Part model, mm, in its own coordinate system. Face numbers are marked on the shaded views. A direction names the side the tool comes from. Round coordinates to 2 decimals unless told otherwise and drop trailing zeros. Write each loop counter-clockwise with the first axis right and the second up, starting at its lowest first coordinate (ties: lowest second). Pieces come first, ordered by that corner, then holes. Notation, with made-up numbers: M -30,23 L 12,23 A21 ccw 12,27 Z; hole C 50.25,-26.75 d7. An arc over 180 degrees is marked long. Use a Markdown table: item, result. Add a question column.
1) Wall check: probe 1 along Z at (x, y) = (12.5, 1); probe 2 along Z at (x, y) = (-1, 12.5); probe 3 along Z at (x, y) = (-0.5, 3.5). Give the ranges that are in metal, low to high.
2) Slice it at B-B on x = 12. Give the number of separate pieces and of enclosed holes in the cut face, plus the area to 3 significant figures.
3) Slice it at A-A on y = 0. Write the cut outline in (x, z).
4) Drop flat-ended pins along their axis: P1, Ø8, axis at x = -9, z = 7, coming from the +Y side; P2, Ø8, axis at x = 7, z = 5, coming from the -Y side; P3, Ø8, axis at x = 2.5, z = 6, coming from the -Y side; P4, Ø6, axis at x = -6.5, y = 3, coming from the -Z side. Give the stop position or say it passes through.
5) Which spindle directions (+Z, -Z, +X, -X, +Y, -Y) get a long thin tool onto all of the face, cutting with end or side? Do the marked faces 1 and 2. Say none if no direction does.
6) Two-plate mould, pull along Y, no slides. Class the marked faces 3, 4 and 5: released by +Y, released by -Y, zero draft, split by the parting line, or undercut.
```python
from build123d import *

# Parameters (mm, degrees)
F0_R     = 15
F1_DEPTH = 14
F2_SIZE  = 1
F3_R     = 11
F4_DEPTH = 4.4
F10_D    = 8
F13_D    = 3


with BuildPart() as f1:
    # F0 (on Top) → F1 (new body)
    with BuildSketch(Plane.XY):
        Circle(F0_R)
    extrude(amount=F1_DEPTH)

    # F2
    f2_edges = [f1.edges().sort_by_distance(p)[0] for p in [
        (-15, 0, 14),
        (-15, 0, 0),
    ]]
    chamfer(f2_edges, length=F2_SIZE)

    # F3 (on Top) → F4 (cut)
    with BuildSketch(Plane.XY):
        Circle(F3_R)
    extrude(amount=F4_DEPTH, mode=Mode.SUBTRACT)

    # F5 (on Front) → F6 (revolve, cut)
    with BuildSketch(Plane.XZ):
        Polygon((14, 4.4), (11, 4.4), (11, 1), (13.05913, 1), align=None)
    revolve(axis=Axis((0, 0, 2.2), (0, 0, 1)), mode=Mode.SUBTRACT)

    # F10 (through all)
    with Locations(Plane(origin=(0, 0, 0), x_dir=(0.707107, 0, 0.707107), z_dir=(0.707107, 0, -0.707107))):
        with Locations((0, 0)):
            Hole(F10_D / 2)

    # F13 (through all)
    with Locations(Plane(origin=(1.5, 0, 1.5), x_dir=(0.707107, 0, -0.707107), z_dir=(-0.707107, 0, -0.707107))):
        with Locations((2.12132, 0)):
            Hole(F13_D / 2)


solid = f1.part
```
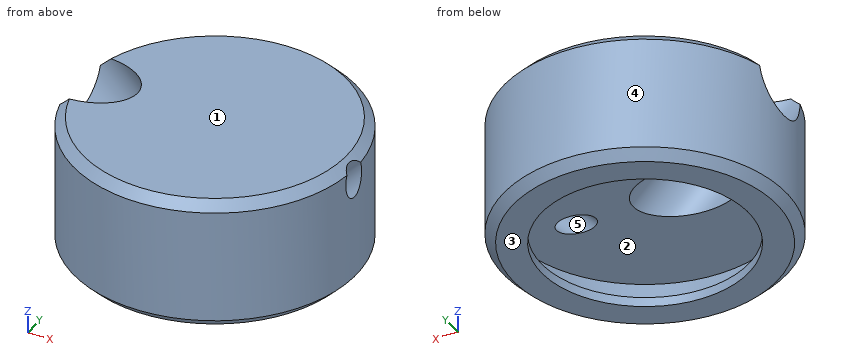
Entries:
| question | item | result |
|---|---|---|
| 1 | probe 1 | z = 0 to 1, 4.4 to 7.92, 11.08 to 14 |
| 1 | probe 2 | z = 0 to 1, 4.4 to 14 |
| 1 | probe 3 | z = 4.4 to 14 |
| 2 | separate pieces | 1 |
| 2 | enclosed holes | 2 |
| 2 | area | 196 mm^2 |
| 3 | outline | M -15,1 L -14,0 L -11,0 L -11,1 L -13.06,1 L -14,4.4 L -10.06,4.4 L -15,9.34 Z; M -8.34,14 L 1.26,4.4 L 5.28,4.4 L 14.44,13.56 L 14,14 Z; M 9.52,4.4 L 14,4.4 L 13.06,1 L 11,1 L 11,0 L 14,0 L 15,1 L 15,9.88 Z |
| 4 | P1 | stops at y = 14.14 |
| 4 | P2 | stops at y = -14.7 |
| 4 | P3 | stops at y = -15 |
| 4 | P4 | stops at z = 4.4 |
| 5 | face 1 | +Z, +X, -X, +Y, -Y |
| 5 | face 2 | none |
| 6 | face 3 | zero draft |
| 6 | face 4 | split by the parting line |
| 6 | face 5 | undercut |
